Study the drawing (mm; zero at the part's minimum x, y, z) and answer. A direction names the side the tool comes from. Coordinates: 2 decimals unless noted, no trailing zeros. Order: outer loops, then holes, each group sorted by start corner. A loop starts at its lowest first (then second) coordinate and runs counter-clockwise, first axis right, second up. Notation, with made-up numbers: (-4.75, 67.5) -> (32.25, 67.5) arc R22 cw to (32.25, 82.5) -> close; hole circle Ø7 at (70, -3.5). An arc over 180 degrees is marked (long way). Answer in a Markdown table with one row per item. Add a question column.
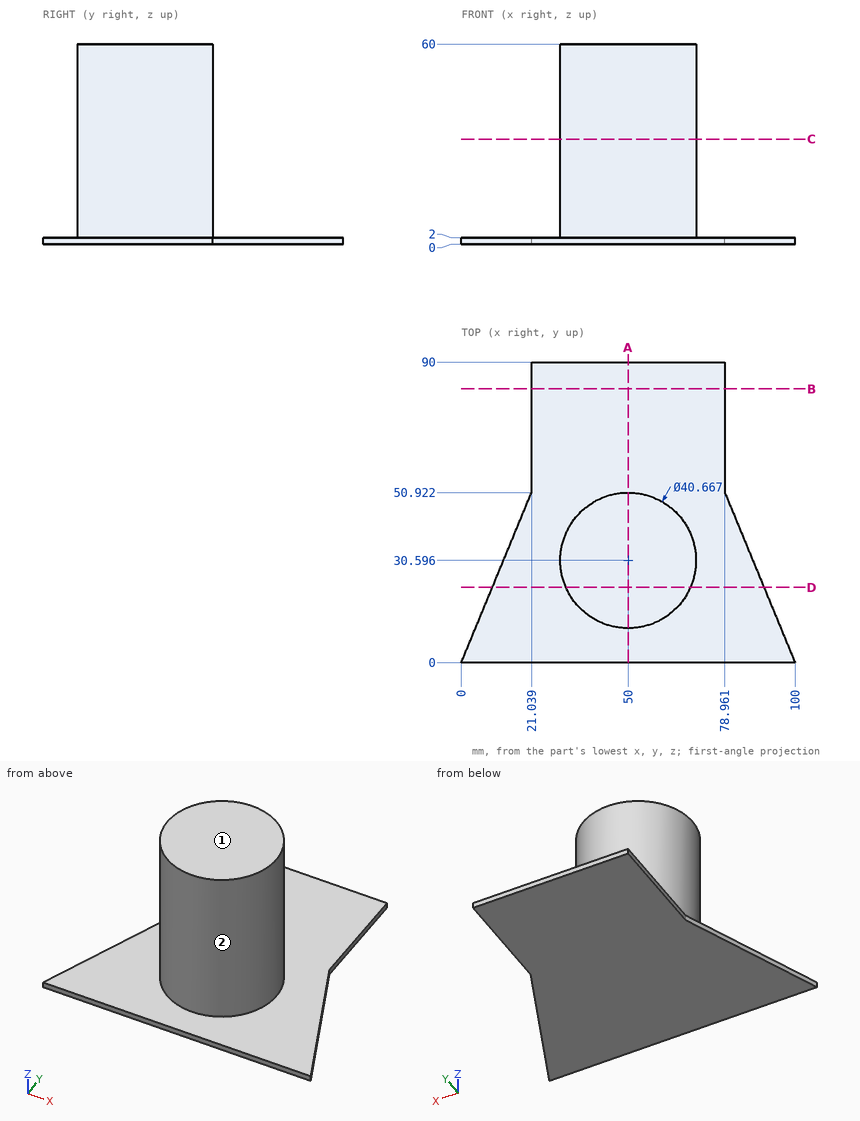
Q1. A cutting plane is placed at B-B (y = 82). Determine the outline of the cut face in (x, z), then the cut area to 3 significant figures.
Q2. Given pin 1 (1 mm diameter, centred on y = 39.5, z = 28.5, fed in from +X); pin 2 (1 mm diameter, centred on y = 21, z = 28, fed in from +X); pin 3 (1 mm diameter, centred on x = 52, z = 51.5, fed in from +Y), each flat-ended and moving along its own axis, determine where each tip first touches the part or whether it passes through.
Q3. A cutting plane is placed at D-D (y = 22.5). Determine the outline of the cut face in (x, z).
Q4. Straight lines are drawn through the part: line 1 (Z direction, x = 69.5, y = 16); line 2 (X direction, y = 38.5, z = 19.5) (1 decimal); line 3 (X direction, y = 24, z = 54). For each, find the intervals that lie inside material, in ascending order.
Q5. A cutting plane is placed at A-A (x = 50). Determine the outline of the cut face in (y, z), then the cut area to 3 significant figures.
Q6. A cutting plane is placed at C-C (z = 31.5). Determine the outline of the cut face in (x, y), then the cut area to 3 significant figures.
Q7. For the marked faces 1 and 2, determine the directions among +Z, -Z, +X, -X, +Y, -Y from which every point of the face is accessible in a straight line to the end or side of a thin tool.
Returned:
| question | item | result |
|---|---|---|
| 1 | outline | (21.04, 0) -> (78.96, 0) -> (78.96, 2) -> (21.04, 2) -> close |
| 1 | area | 116 mm² |
| 2 | pin 1 | stops at x = 68.52 |
| 2 | pin 2 | stops at x = 68.19 |
| 2 | pin 3 | stops at y = 50.87 |
| 3 | outline | (9.3, 0) -> (90.7, 0) -> (90.7, 2) -> (68.65, 2) -> (68.65, 60) -> (31.35, 60) -> (31.35, 2) -> (9.3, 2) -> close |
| 4 | line 1 | z = 0 to 2 |
| 4 | line 2 | x = 31.3 to 68.7 |
| 4 | line 3 | x = 30.77 to 69.23 |
| 5 | outline | (0, 0) -> (90, 0) -> (90, 2) -> (50.93, 2) -> (50.93, 60) -> (10.26, 60) -> (10.26, 2) -> (0, 2) -> close |
| 5 | area | 2,540 mm² |
| 6 | outline | circle Ø40.67 at (50, 30.6) |
| 6 | area | 1,300 mm² |
| 7 | face 1 | +Z, +X, -X, +Y, -Y |
| 7 | face 2 | +Z |
